Model file for the job. Use its own axes, mm. Give positions to 0.01 mm unless a question says otherwise; leave off trailing zeros. Loops run counter-clockwise (first coordinate to the right, second up) from the corner with the lowest first, then second, coordinate; pieces in that order, holes last. Notation, with made-up numbers: M -6.75,48 L 4.25,48 A10 cw 4.25,57 Z; hole C 55.5,1.25 d6. An arc over 180 degrees is marked long. Answer in a Markdown table with one row per item.
```python
from build123d import *

# Parameters (mm, degrees)
ESBO_O1_R                = 1.55
ESBO_O1_W                = 10
ESBO_O1_H                = 3.2
RESSALTO_EXTRUS_O1_DEPTH = 3
ESBO_O2_R                = 1.55
CORTE_EXTRUS_O1_DEPTH    = 177.666352201
ESBO_O3_R                = 1.55
CORTE_EXTRUS_O2_DEPTH    = 10


with BuildPart() as part:
    # Esboço1 → Ressalto-extrusão1 (new body)
    with BuildSketch(Plane.XY):
        with BuildLine():
            Line((0, 82), (0, 135))
            Line((0, 135), (2, 139))
            Line((2, 139), (107, 139))
            Line((107, 139), (109, 135))
            Line((109, 135), (109, 82))
            Line((109, 82), (91, 82))
            Line((91, 82), (89.5, 80.5))
            Line((89.5, 80.5), (89.5, 11.5))
            ThreePointArc((89.5, 11.5), (89.939339828, 10.439339828), (91, 10))
            Line((91, 10), (93, 10))
            Line((93, 10), (95, 8))
            Line((95, 8), (109, 8))
            Line((109, 8), (109, 3))
            ThreePointArc((109, 3), (108.121320344, 0.878679656), (106, 0))
            Line((106, 0), (3, 0))
            ThreePointArc((3, 0), (0.878679656, 0.878679656), (0, 3))
            Line((0, 3), (0, 8))
            Line((0, 8), (14, 8))
            Line((14, 8), (16, 10))
            Line((16, 10), (18, 10))
            ThreePointArc((18, 10), (19.060660172, 10.439339828), (19.5, 11.5))
            Line((19.5, 11.5), (19.5, 80.5))
            Line((19.5, 80.5), (18, 82))
            Line((18, 82), (0, 82))
        make_face()
        with Locations((38.75, 4.6)):
            Circle(ESBO_O1_R, mode=Mode.SUBTRACT)
        with Locations((70.25, 4.6)):
            Circle(ESBO_O1_R, mode=Mode.SUBTRACT)
        with Locations((54.5, 85)):
            Circle(ESBO_O1_R, mode=Mode.SUBTRACT)
        with Locations((6, 124)):
            Circle(ESBO_O1_R, mode=Mode.SUBTRACT)
        with Locations((103, 124)):
            Circle(ESBO_O1_R, mode=Mode.SUBTRACT)
        with Locations((23, 4.6)):
            Rectangle(ESBO_O1_W, ESBO_O1_H, mode=Mode.SUBTRACT)
        with Locations((54.5, 4.6)):
            Rectangle(ESBO_O1_W, ESBO_O1_H, mode=Mode.SUBTRACT)
        with Locations((86, 4.6)):
            Rectangle(ESBO_O1_W, ESBO_O1_H, mode=Mode.SUBTRACT)
        with BuildLine():
            Line((26.5, 13.1), (51.5, 13.1))
            ThreePointArc((51.5, 13.1), (53.05, 11.55), (51.5, 10))
            Line((51.5, 10), (26.5, 10))
            ThreePointArc((26.5, 10), (24.95, 11.55), (26.5, 13.1))
        make_face(mode=Mode.SUBTRACT)
        with BuildLine():
            Line((57.5, 13.1), (82.5, 13.1))
            ThreePointArc((82.5, 13.1), (84.05, 11.55), (82.5, 10))
            Line((82.5, 10), (57.5, 10))
            ThreePointArc((57.5, 10), (55.95, 11.55), (57.5, 13.1))
        make_face(mode=Mode.SUBTRACT)
    extrude(amount=RESSALTO_EXTRUS_O1_DEPTH)

    # Esboço2 → Corte-extrusão1 (cut, through all)
    with BuildSketch(Plane.XY.offset(3)):
        with Locations((47, 117)):
            Circle(ESBO_O2_R)
        with Locations((47, 125)):
            Circle(ESBO_O2_R)
        with Locations((62, 117)):
            Circle(ESBO_O2_R)
        with Locations((62, 125)):
            Circle(ESBO_O2_R)
        with BuildLine():
            Line((47, 24.1), (62, 24.1))
            ThreePointArc((62, 24.1), (65, 21.1), (62, 18.1))
            Line((62, 18.1), (47, 18.1))
            ThreePointArc((47, 18.1), (44, 21.1), (47, 24.1))
        make_face()
        with BuildLine():
            Line((21.05, 129), (21.05, 89))
            ThreePointArc((21.05, 89), (19.5, 87.45), (17.95, 89))
            Line((17.95, 89), (17.95, 129))
            ThreePointArc((17.95, 129), (19.5, 130.55), (21.05, 129))
        make_face()
        with BuildLine():
            Line((29.7, 18.1), (29.7, 48.1))
            ThreePointArc((29.7, 48.1), (31.25, 49.65), (32.8, 48.1))
            Line((32.8, 48.1), (32.8, 18.1))
            ThreePointArc((32.8, 18.1), (31.25, 16.55), (29.7, 18.1))
        make_face()
        with BuildLine():
            Line((75.9, 96.1), (75.9, 66.1))
            ThreePointArc((75.9, 66.1), (74.35, 64.55), (72.8, 66.1))
            Line((72.8, 66.1), (72.8, 96.1))
            ThreePointArc((72.8, 96.1), (74.35, 97.65), (75.9, 96.1))
        make_face()
        with BuildLine():
            Line((48, 96.1), (48, 66.1))
            ThreePointArc((48, 66.1), (46.45, 64.55), (44.9, 66.1))
            Line((44.9, 66.1), (44.9, 96.1))
            ThreePointArc((44.9, 96.1), (46.45, 97.65), (48, 96.1))
        make_face()
        with BuildLine():
            Line((28, 118.5), (40, 118.5))
            ThreePointArc((40, 118.5), (43.5, 115), (40, 111.5))
            Line((40, 111.5), (28, 111.5))
            ThreePointArc((28, 111.5), (24.5, 115), (28, 118.5))
        make_face()
        with BuildLine():
            Line((28, 130.5), (40, 130.5))
            ThreePointArc((40, 130.5), (43.5, 127), (40, 123.5))
            Line((40, 123.5), (28, 123.5))
            ThreePointArc((28, 123.5), (24.5, 127), (28, 130.5))
        make_face()
        with BuildLine():
            Line((91.05, 129), (91.05, 89))
            ThreePointArc((91.05, 89), (89.5, 87.45), (87.95, 89))
            Line((87.95, 89), (87.95, 129))
            ThreePointArc((87.95, 129), (89.5, 130.55), (91.05, 129))
        make_face()
        with BuildLine():
            Line((69, 118.5), (81, 118.5))
            ThreePointArc((81, 118.5), (84.5, 115), (81, 111.5))
            Line((81, 111.5), (69, 111.5))
            ThreePointArc((69, 111.5), (65.5, 115), (69, 118.5))
        make_face()
        with BuildLine():
            Line((69, 130.5), (81, 130.5))
            ThreePointArc((81, 130.5), (84.5, 127), (81, 123.5))
            Line((81, 123.5), (69, 123.5))
            ThreePointArc((69, 123.5), (65.5, 127), (69, 130.5))
        make_face()
        with BuildLine():
            Line((39.5, 32.65), (79.5, 32.65))
            ThreePointArc((79.5, 32.65), (81.05, 31.1), (79.5, 29.55))
            Line((79.5, 29.55), (39.5, 29.55))
            ThreePointArc((39.5, 29.55), (37.95, 31.1), (39.5, 32.65))
        make_face()
        with BuildLine():
            Line((39.5, 57.65), (79.5, 57.65))
            ThreePointArc((79.5, 57.65), (81.05, 56.1), (79.5, 54.55))
            Line((79.5, 54.55), (39.5, 54.55))
            ThreePointArc((39.5, 54.55), (37.95, 56.1), (39.5, 57.65))
        make_face()
    extrude(amount=-CORTE_EXTRUS_O1_DEPTH, mode=Mode.SUBTRACT)

    # Esboço3 → Corte-extrusão2 (cut)
    with BuildSketch(Plane.XY.offset(3)):
        with Locations((54.693176617, 134.937304028)):
            Circle(ESBO_O3_R)
        with Locations((9.5, 134.937304028)):
            Circle(ESBO_O3_R)
        with Locations((99.5, 134.937304028)):
            Circle(ESBO_O3_R)
    extrude(amount=-CORTE_EXTRUS_O2_DEPTH, mode=Mode.SUBTRACT)


solid = part.part
```
(1) Flat gauge pins, fed straight in: P1, Ø1.5, axis at y = 29, z = 1.5, coming from the +X side; P2, Ø2.5, axis at x = 38.75, y = 4.6, coming from the -Z side. Where does each tip first touch, or does it go through?
Established:
| item | result |
|---|---|
| P1 | stops at x = 89.5 |
| P2 | passes through |
(2) Mould opens along X. For faces 1 (the flat face through (102, 8, 1)), 2 (the flat face through (109, 6, 1)), 3 (the flat face through (32.8, 33, 2)), 4 (the flat face through (0, 108, 1)) say: pulls with the +X half, pulls with the -X half, needs draft (parallel to the pull), parting line crosses it, or undercut.
Established:
| item | result |
|---|---|
| face 1 | needs draft |
| face 2 | pulls with the +X half |
| face 3 | undercut |
| face 4 | pulls with the -X half |
(3) Saw through at B-B, the plane y = 31.1. Give the cut face in (x, z), and give its area (3 significant figures).
Established:
| item | result |
|---|---|
| outline | M 19.5,0 L 29.7,0 L 29.7,3 L 19.5,3 Z; M 32.8,0 L 37.95,0 L 37.95,3 L 32.8,3 Z; M 81.05,0 L 89.5,0 L 89.5,3 L 81.05,3 Z |
| area | 71.4 mm2 |
(4) Saw through at A-A, the plane x = 6. Give the cut face in (y, z), and give its area (3 significant figures).
Established:
| item | result |
|---|---|
| outline | M 0,0 L 8,0 L 8,3 L 0,3 Z; M 82,0 L 122.45,0 L 122.45,3 L 82,3 Z; M 125.55,0 L 139,0 L 139,3 L 125.55,3 Z |
| area | 186 mm2 |
(5) Wall check: L1, parallel to X at y = 121, z = 0.4; L2, parallel to Y at x = 9.5, z = 0.9. Give the ranges that are in metal, low to high.
Established:
| item | result |
|---|---|
| L1 | x = 0 to 17.95, 21.05 to 87.95, 91.05 to 109 |
| L2 | y = 0 to 8, 82 to 133.39, 136.49 to 139 |
(6) Saw through at C-C, the plane z = 2.3. Count the separate pieces of the cut face and the enclosed holes in it, and give its area (3 significant figures).
Established:
| item | result |
|---|---|
| separate pieces | 1 |
| enclosed holes | 29 |
| area | 10,500 mm2 |
